Input: part model. Units: mm. Frame: model coordinates. Face numbers are marked on the shaded views. A direction names the side the tool comes from. Round coordinates to 2 decimals unless told otherwise and drop trailing zeros. Loops run counter-clockwise (first coordinate to the right, second up) from the corner with the lowest first, then second, coordinate; pieces in that order, holes last. Notation, with made-up numbers: (54, -12) - (112, -12) arc R10 ccw to (112, 6) - close; hole circle Ø8 at (-10.75, 48). An arc over 180 degrees is marked (long way). Write each question's results on one line, items separated by ' | '.
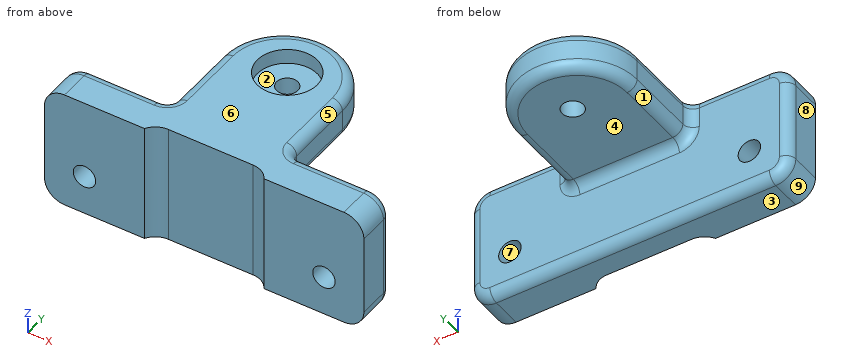
from build123d import *

# Parameters (mm, degrees)
SKETCH1_W                                = 101.6
SKETCH1_H                                = 38.1
BASEPLATE_DEPTH                          = 12.7
VERTBOSS_DEPTH                           = 12.7
F_9_32_0_28125_DIAMETER_HOLE1_D          = 7.14375
CBORE_FOR_1_4_HEX_HEAD_BOLT1_D           = 6.7564
CBORE_FOR_1_4_HEX_HEAD_BOLT1_CBORE_D     = 19.05
CBORE_FOR_1_4_HEX_HEAD_BOLT1_CBORE_DEPTH = 4.7752
SKETCH11_W                               = 38
SKETCH11_H                               = 3.17
BOTTOMSLOT_DEPTH                         = 123.615578129
FILLET1_R                                = 6.35
FILLET2_R                                = 3.17


with BuildPart() as part:
    # Sketch1 → BasePlate (new body)
    with BuildSketch(Plane(origin=(0, 0, 0), x_dir=(1, 0, 0), z_dir=(0, 1, 0))):
        with Locations((50.8, 19.05)):
            Rectangle(SKETCH1_W, SKETCH1_H)
    extrude(amount=BASEPLATE_DEPTH)

    # Sketch3 → VertBoss (add)
    with BuildSketch(Plane.XY):
        with BuildLine():
            Line((31.8, 0), (31.8, 38.1))
            ThreePointArc((31.8, 38.1), (50.8, 57.1), (69.8, 38.1))
            Line((69.8, 38.1), (69.8, 0))
            Line((69.8, 0), (31.8, 0))
        make_face()
    extrude(amount=-VERTBOSS_DEPTH)

    # 9/32 (0.28125) Diameter Hole1 (through all)
    with Locations(Plane(origin=(0, 12.7, 0), x_dir=(1, 0, 0), z_dir=(0, 1, 0))):
        with Locations((88.9, 25.4), (12.7, 25.4)):
            Hole(F_9_32_0_28125_DIAMETER_HOLE1_D / 2)

    # CBORE for 1/4 Hex Head Bolt1 (through all)
    with Locations(Plane.XY):
        with Locations((50.8, 40.318171365)):
            CounterBoreHole(CBORE_FOR_1_4_HEX_HEAD_BOLT1_D / 2, CBORE_FOR_1_4_HEX_HEAD_BOLT1_CBORE_D / 2, CBORE_FOR_1_4_HEX_HEAD_BOLT1_CBORE_DEPTH)

    # Sketch11 → BottomSlot (cut, through all)
    with BuildSketch(Plane.XY):
        with Locations((50.8, 1.585)):
            Rectangle(SKETCH11_W, SKETCH11_H)
    extrude(amount=-BOTTOMSLOT_DEPTH, mode=Mode.SUBTRACT)

    # Fillet1
    # the kernel refuses this fillet: 6.35 mm, written as the material it adds along each edge
    with BuildSketch(Plane(origin=(69.8, 3.17, 0), x_dir=(-1, 0, 0), z_dir=(0, 0, -1))) as fillet1_piece_1:
        with BuildLine():
            CenterArc((5.49637153, -6.35), FILLET1_R, 90, 59.947892244)
            Line((0, -3.17), (0, 0))
            Line((0, 0), (5.49637153, 0))
        make_face()
    extrude(amount=38.1)
    with BuildSketch(Plane(origin=(31.8, 3.17, 0), x_dir=(0, -1, 0), z_dir=(0, 0, -1))) as fillet1_piece_2:
        with BuildLine():
            CenterArc((6.35, -5.49637153), FILLET1_R, 120.052107756, 59.947892244)
            Line((0, -5.49637153), (0, 0))
            Line((0, 0), (3.17, 0))
        make_face()
    extrude(amount=38.1)
    # the kernel refuses this fillet: 6.35 mm, written as the material it takes off along each edge
    with BuildSketch(Plane(origin=(0, -15.875, -38.1), x_dir=(0, 0, 1), z_dir=(0, 1, 0)), Plane(origin=(0, -15.875, 0), x_dir=(1, 0, 0), z_dir=(0, 1, 0))) as fillet1_2_piece_1:
        with BuildLine():
            CenterArc((FILLET1_R, FILLET1_R), FILLET1_R, 180, 90)
            Line((0, FILLET1_R), (0, 0))
            Line((0, 0), (FILLET1_R, 0))
        make_face()
    extrude(amount=44.45, mode=Mode.SUBTRACT)
    with BuildSketch(Plane(origin=(101.6, -15.875, -38.1), x_dir=(0, 0, 1), z_dir=(0, 1, 0)), Plane(origin=(101.6, -15.875, 0), x_dir=(-1, 0, 0), z_dir=(0, 1, 0))) as fillet1_2_piece_2:
        with BuildLine():
            CenterArc((FILLET1_R, -FILLET1_R), FILLET1_R, 90, 90)
            Line((0, -FILLET1_R), (0, 0))
            Line((0, 0), (FILLET1_R, 0))
        make_face()
    extrude(amount=44.45, mode=Mode.SUBTRACT)

    # Fillet2
    fillet2_edges = [part.edges().sort_by_distance(p)[0] for p in [
        (82.525, 12.7, 0),
        (31.8, 25.4, -12.7),
        (69.8, 25.4, -12.7),
        (31.8, 25.4, 0),
        (69.8, 25.4, 0),
        (50.8, 57.1, 0),
        (31.8, 12.7, -6.35),
        (50.8, 57.1, -12.7),
        (69.8, 12.7, -6.35),
        (50.8, 12.7, -12.7),
        (0, 12.7, -19.05),
        (50.8, 12.7, -38.1),
        (19.075, 12.7, 0),
        (101.6, 12.7, -19.05),
        (99.740128061, 12.7, -1.859871939),
        (99.740128061, 12.7, -36.240128061),
        (1.859871939, 12.7, -1.859871939),
        (1.859871939, 12.7, -36.240128061),
    ]]
    fillet(fillet2_edges, radius=FILLET2_R)


solid = part.part
1. Section query B-B, the plane y = 35. Output: boundary loops of the cut face in (x, z), plus the area to 3 significant figures.
Answer:
outline: (31.8, -9.53) arc R3.17 ccw to (34.97, -12.7) - (66.63, -12.7) arc R3.17 ccw to (69.8, -9.53) - (69.8, -3.17) arc R3.17 ccw to (66.63, 0) - (58.7, 0) - (58.7, -4.78) - (42.9, -4.78) - (42.9, 0) - (34.97, 0) arc R3.17 ccw to (31.8, -3.17) - close | area: 399 mm^2
2. Section query C-C, the plane z = -8. Output: boundary loops of the cut face in (x, y), plus the area to 3 significant figures.
Answer:
outline: (0, 0) - (31.8, 0) arc R6.35 cw to (37.3, 3.17) - (64.3, 3.17) arc R6.35 cw to (69.8, 0) - (101.6, 0) - (101.6, 9.53) arc R3.17 ccw to (98.43, 12.7) - (72.97, 12.7) arc R3.17 cw to (69.8, 15.87) - (69.8, 38.1) arc R19 ccw to (31.8, 38.1) - (31.8, 15.87) arc R3.17 cw to (28.63, 12.7) - (3.17, 12.7) arc R3.17 ccw to (0, 9.53) - close; hole circle Ø6.76 at (50.8, 40.32) | area: 2,680 mm^2
3. Set-up query: the marked faces 1, 2, 3, 4 and 5. Return all of +Z, -Z, +X, -X, +Y, -Y with unobstructed straight access to the full face (end or side cutting, diameter ignored); none if empty.
Answer:
face 1: -Z, -X, +Y | face 2: +Z | face 3: -Z, +X, -X, +Y, -Y | face 4: -Z, +X, -X, +Y | face 5: +Z, +X, +Y
4. Mould query, pull axis Z, two halves, no side actions, for the marked faces 6, 7, 8 and 9. Classes: pulls with the +Z half, pulls with the -Z half, needs draft (parallel to the pull), parting line crosses it, or undercut.
Answer:
face 6: pulls with the +Z half | face 7: undercut | face 8: needs draft | face 9: pulls with the -Z half
5. Section query D-D, the plane x = 50.8. Output: boundary loops of the cut face in (y, z), plus the area to 3 significant figures.
Answer:
outline: (3.17, -38.1) - (9.53, -38.1) arc R3.17 ccw to (12.7, -34.93) - (12.7, -15.87) arc R3.17 cw to (15.87, -12.7) - (36.94, -12.7) - (36.94, -4.78) - (30.79, -4.78) - (30.79, 0) - (3.17, 0) - close; (43.7, -12.7) - (53.93, -12.7) arc R3.17 ccw to (57.1, -9.53) - (57.1, -3.17) arc R3.17 ccw to (53.93, 0) - (49.84, 0) - (49.84, -4.78) - (43.7, -4.78) - close | area: 778 mm^2
6. Section query A-A, the plane x = 88.9. Output: boundary loops of the cut face in (y, z).
Answer:
outline: (0, -38.1) - (9.53, -38.1) arc R3.17 ccw to (12.7, -34.93) - (12.7, -28.97) - (0, -28.97) - close; (0, -21.83) - (12.7, -21.83) - (12.7, -3.17) arc R3.17 ccw to (9.53, 0) - (0, 0) - close
7. Line query: line 1 (X direction, y = 8, z = -25); line 2 (X direction, y = 5.5, z = -25.4); line 3 (Y direction, x = 28, z = -7.5). Output: solid intervals per line, ascending. Write a range as [from, to].
Answer:
line 1: [0, 9.15], [16.25, 85.35], [92.45, 101.6] | line 2: [0, 9.13], [16.27, 85.33], [92.47, 101.6] | line 3: [0, 12.7]
8. Contact query for flat-ended pins moving along their axis: pin 1 (25 mm diameter, centred on x = 50.8, y = 40.32, fed in from -Z); pin 2 (10 mm diameter, centred on x = 13.5, z = -17, fed in from +Y); pin 3 (6 mm diameter, centred on x = 87, y = 13, fed in from +Z); pin 4 (9.5 mm diameter, centred on x = 88.9, z = -25.4, fed in from -Y). Output: stop coordinate, or through.
Answer:
pin 1: z = -12.7 | pin 2: y = 12.7 | pin 3: z = -0.04 | pin 4: y = 0
